from build123d import *

# Parameters (mm, degrees)
SKETCH1_W           = 28
SKETCH1_H           = 68
BOSS_EXTRUDE1_DEPTH = 1.25
SKETCH7_W           = 28
SKETCH7_H           = 68
SKETCH7_W_2         = 25.5
SKETCH7_H_2         = 65.5
BOSS_EXTRUDE4_DEPTH = 7.75
SKETCH18_W          = 11
SKETCH18_H          = 2.7
CUT_EXTRUDE10_DEPTH = 1.25
SKETCH13_R          = 1.05
BOSS_EXTRUDE7_DEPTH = 5
LPATTERN2_COUNT     = 4
LPATTERN2_PITCH     = 5
SKETCH14_W          = 10
SKETCH14_H          = 5
CUT_EXTRUDE5_DEPTH  = 5
FILLET1_R           = 1
SKETCH6_R           = 1.25
BOSS_EXTRUDE3_DEPTH = 4
FILLET3_R           = 5
FILLET4_R           = 1
FILLET7_R           = 1


with BuildPart() as part:
    # Sketch1 → Boss-Extrude1 (new body)
    with BuildSketch(Plane.XY):
        with Locations((-2.825688073, -2.660550459)):
            Rectangle(SKETCH1_W, SKETCH1_H)
    extrude(amount=BOSS_EXTRUDE1_DEPTH)

    # Sketch7 → Boss-Extrude4 (add)
    with BuildSketch(Plane.XY.offset(1.25)):
        with Locations((-2.825688073, -2.660550459)):
            Rectangle(SKETCH7_W, SKETCH7_H)
        with Locations((-2.825688073, -2.660550459)):
            Rectangle(SKETCH7_W_2, SKETCH7_H_2, mode=Mode.SUBTRACT)
    extrude(amount=BOSS_EXTRUDE4_DEPTH)

    # Sketch18 → Cut-Extrude10 (cut)
    with BuildSketch(Plane(origin=(0, 31.339449541, 0), x_dir=(1, 0, 0), z_dir=(0, 1, 0))):
        with Locations((-2.825688073, -4.9)):
            Rectangle(SKETCH18_W, SKETCH18_H)
    extrude(amount=-CUT_EXTRUDE10_DEPTH, mode=Mode.SUBTRACT)

    # Sketch13 → Boss-Extrude7 (add)
    with BuildSketch(Plane.XZ.offset(36.660550459)):
        with BuildLine():
            Line((12.674311927, 7.5), (11.174311927, 6.303164343))
            Line((11.174311927, 6.303164343), (11.174311927, 9))
            ThreePointArc((11.174311927, 9), (13.734972098, 10.060660172), (12.674311927, 7.5))
        make_face()
        with Locations(Location((12.674311927, 9, 0), (0, 0, 270))):
            Circle(SKETCH13_R, mode=Mode.SUBTRACT)
    boss_extrude7 = extrude(amount=-BOSS_EXTRUDE7_DEPTH)

    # LPattern2: Boss-Extrude7 ×4, 1 skipped
    with Locations(*[(0, i * LPATTERN2_PITCH, 0) for i in range(1, LPATTERN2_COUNT) if i not in (2,)]):
        add(boss_extrude7)

    # Sketch14 → Cut-Extrude5 (cut)
    with BuildSketch(Plane(origin=(11.174311927, 0, 0), x_dir=(0, 0, -1), z_dir=(1, 0, 0))):
        with Locations((-8.964747177, -34.160550459)):
            Rectangle(SKETCH14_W, SKETCH14_H)
    extrude(amount=CUT_EXTRUDE5_DEPTH, mode=Mode.SUBTRACT)

    # Fillet1
    fillet1_edges = [part.edges().sort_by_distance(p)[0] for p in [
        (-2.825688073, 31.339449541, 0),
        (11.174311927, -2.660550459, 0),
        (11.174311927, -36.660550459, 4.5),
        (-2.825688073, -36.660550459, 0),
        (-16.825688073, -2.660550459, 0),
        (-16.825688073, 31.339449541, 4.5),
        (11.174311927, 31.339449541, 4.5),
        (-16.825688073, -36.660550459, 4.5),
    ]]
    fillet(fillet1_edges, radius=FILLET1_R)

    # Sketch6 → Boss-Extrude3 (add)
    # profile 1 of 2: a face of its own
    with BuildSketch(Plane.XY.offset(9)):
        with BuildLine():
            Line((-16.825688073, 1.839449541), (-16.825688073, 17.839449541))
            ThreePointArc((-16.825688073, 17.839449541), (-24.825688073, 9.839449541), (-16.825688073, 1.839449541))
        make_face()
        with Locations((-20.825688073, 9.839449541)):
            Circle(SKETCH6_R, mode=Mode.SUBTRACT)
    # profile 2 of 2: a face of its own
    with BuildSketch(Plane.XY.offset(9)):
        with BuildLine():
            Line((11.174311927, 1.839449541), (11.174311927, 17.839449541))
            ThreePointArc((11.174311927, 17.839449541), (19.174311927, 9.839449541), (11.174311927, 1.839449541))
        make_face()
        with Locations(Location((15.174311927, 9.839449541, 0), (0, 0, 180))):
            Circle(SKETCH6_R, mode=Mode.SUBTRACT)
    extrude(amount=-BOSS_EXTRUDE3_DEPTH)

    # Fillet3
    fillet3_edges = [part.edges().sort_by_distance(p)[0] for p in [
        (-16.825688073, 1.839449541, 7),
        (-16.825688073, 17.839449541, 7),
        (11.174311927, 17.839449541, 7),
        (11.174311927, 1.839449541, 7),
    ]]
    fillet(fillet3_edges, radius=FILLET3_R)

    # Fillet4
    fillet4_edges = [part.edges().sort_by_distance(p)[0] for p in [
        (-16.825688073, 9.839449541, 5),
        (11.174311927, 9.839449541, 5),
    ]]
    fillet(fillet4_edges, radius=FILLET4_R)

    # Fillet7
    fillet7_edges = [part.edges().sort_by_distance(p)[0] for p in [
        (2.674311927, 31.339449541, 4.9),
        (-2.825688073, 31.339449541, 3.55),
        (-8.325688073, 31.339449541, 4.9),
        (-2.825688073, 31.339449541, 6.25),
    ]]
    fillet(fillet7_edges, radius=FILLET7_R)


solid = part.part
Design review of the part built by this model. Coordinates are the model's own, in mm. A direction names the side the tool comes from. Round coordinates to 2 decimals unless told otherwise and drop trailing zeros. Write each loop counter-clockwise with the first axis right and the second up, starting at its lowest first coordinate (ties: lowest second). Pieces come first, ordered by that corner, then holes.
Item 1: Consider section B-B on y = -26. Give the boundary of the cut face in (x, z), and give its area (3 significant figures).
Item 2: Consider section A-A on x = 15. Give the boundary of the cut face in (y, z).
Item 3: For pin 1 Ø1 at (y, z) = (-19, 2.5) entering from -X; pin 2 Ø3.5 at (x, y) = (-19.5, 11.5) entering from -Z; pin 3 Ø6 at (x, z) = (-19.5, 9) entering from -Y, all flat-tipped, find the tip position at first contact; note any pin that passes through.
Item 4: For faces 5 (the flat face through (11.935, -29.196, 6.91)), 6 (the flat face through (-15.576, -3, 5)), 7 (the cylindrical face through (13.699, -29.196, 10.095)), 8 (the flat face through (12, -16.661, 8)), 9 (the flat face through (11.174, -10, 4)), list the 3-axis set-ups (+Z, -Z, +X, -X, +Y, -Y) from which the entire face can be reached by the end or side of a thin tool; tool diameter is ignored.
Item 5: Wall thickness on L1, parallel to X at y = 26, z = 3.25; L2, parallel to Y at x = 7, z = 8; L3, parallel to X at y = -27, z = 8.25: over which ranges is each line inside the solid? List them lowest first.
Item 6: Draft analysis for pull direction Y (two halves, no side actions). For faces 1 (the cylindrical face through (11.74, -29.2, 8.52)), 2 (the flat face through (-3, 30.089, 3)), 3 (the flat face through (12, -21.661, 8)), 4 (the flat face through (12, -31.661, 8)), state which applies: released by +Y, released by -Y, zero draft, split by the parting line, or undercut.
Item 7: Consider section C-C on y = 13. Give the boundary of the cut face in (x, z).
Check values:
1. outline: (-16.83, 1) arc R1 ccw to (-15.83, 0) - (10.17, 0) arc R1 ccw to (11.17, 1) - (11.17, 9) - (9.92, 9) - (9.92, 1.25) - (-15.58, 1.25) - (-15.58, 9) - (-16.83, 9) - close
1. area: 53.9 mm2
2. outline: (2.81, 5) - (8.6, 5) - (8.6, 9) - (2.81, 9) - close; (11.08, 5) - (16.87, 5) - (16.87, 9) - (11.08, 9) - close
3. pin 1: stops at x = -16.83
3. pin 2: stops at z = 5
3. pin 3: stops at y = -36.4
4. face 5: -Z, +X, -Y
4. face 6: +Z
4. face 7: -Y
4. face 8: +Z, -Z, +X
4. face 9: -Z, +X
5. L1: x = -16.83 to -15.58, 9.92 to 11.17
5. L2: y = -36.66 to -35.41, 30.09 to 31.34
5. L3: x = -16.83 to -15.58, 9.92 to 11.94, 13.41 to 13.97
6. face 1: zero draft
6. face 2: undercut
6. face 3: undercut
6. face 4: released by -Y
7. outline: (-24.17, 5) - (-17.83, 5) arc R1 cw to (-16.83, 4) - (-16.83, 1) arc R1 ccw to (-15.83, 0) - (10.17, 0) arc R1 ccw to (11.17, 1) - (11.17, 4) arc R1 cw to (12.17, 5) - (18.52, 5) - (18.52, 9) - (9.92, 9) - (9.92, 1.25) - (-15.58, 1.25) - (-15.58, 9) - (-24.17, 9) - close
